Study the drawing (mm; zero at the part's minimum x, y, z) and answer. A direction names the side the tool comes from. Coordinates: 2 decimals unless noted, no trailing zeros. Loops run counter-clockwise (first coordinate to the right, second up) from the corner with the lowest first, then second, coordinate; pieces in that order, holes last. Notation, with made-up numbers: (-13, -21) - (38, -21) arc R21 cw to (38, 10) - close; hole circle Ø2 at (-19.5, -19.5). An arc over 180 degrees is marked (long way). Use one line per item in the form item = value.
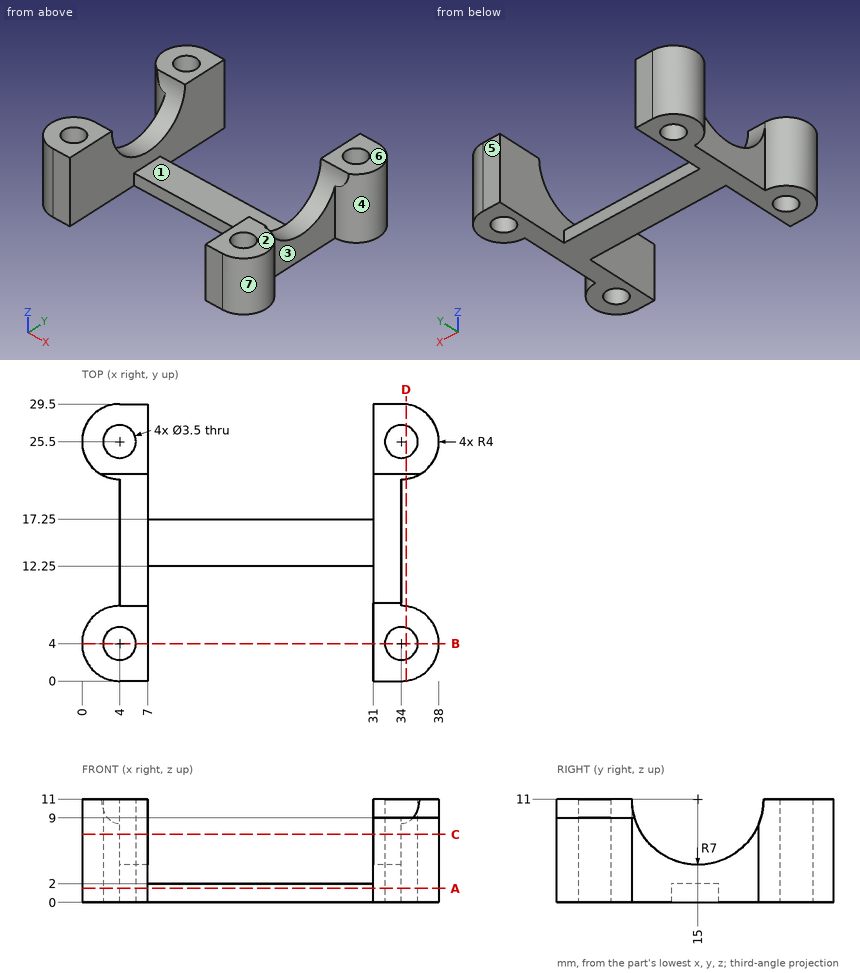
Item 1: The part is cut by section B-B on y = 4. Give the vertices of the cut face in (x, z).
Results below:
outline = (0, 0) - (2.25, 0) - (2.25, 11) - (0, 11) - close; (5.75, 0) - (7, 0) - (7, 11) - (5.75, 11) - close; (31, 0) - (32.25, 0) - (32.25, 9) - (31, 9) - close; (35.75, 0) - (38, 0) - (38, 9) - (35.75, 9) - close
Item 2: Which of the six approach directions +Z, -Z, +X, -X, +Y, -Y give full straight-line access (tool end or side, diameter ignored) to the marked faces 1, 2 and 3?
Results below:
face_1 = +Z, +Y, -Y
face_2 = +Z, +X, -Y
face_3 = +Z, -Z, +X
Item 3: The part is cut by section A-A on z = 1.5. Give the vertices of the cut face in (x, y), plus the area to 3 significant figures.
Results below:
outline = (4, 0) - (7, 0) - (7, 12.25) - (31, 12.25) - (31, 0) - (34, 0) arc R4 ccw to (34, 8) - (34, 21.5) arc R4 ccw to (34, 29.5) - (31, 29.5) - (31, 17.25) - (7, 17.25) - (7, 29.5) - (4, 29.5) arc R4 ccw to (4, 21.5) - (4, 8) arc R4 ccw to start; hole circle Ø3.5 at (4, 4); hole circle Ø3.5 at (4, 25.5); hole circle Ø3.5 at (34, 4); hole circle Ø3.5 at (34, 25.5)
area = 359 mm²
Item 4: Find the intervals of material crossed by L1, parallel to X at y = 26.75, z = 2; L2, parallel to Y at x = 33.5, z = 2.5; L3, parallel to Y at x = 35, z = 3, in increasing order.
Results below:
L1 = 0.2 to 2.78, 5.22 to 7, 31 to 32.78, 35.22 to 37.8
L2 = 0 to 2.32, 5.68 to 23.82, 27.18 to 29.5
L3 = 0.13 to 2.56, 5.44 to 7.87, 21.63 to 24.06, 26.94 to 29.37
Item 5: For a pull along Y with two mould halves and no side action, classify the marked faces 4, 5, 6 and 7 as +Y half, -Y half, draft (parallel to the pull), parting line (faces both ways), or undercut.
Results below:
face_4 = undercut
face_5 = +Y half
face_6 = draft
face_7 = undercut
Item 6: The part is cut by section D-D on x = 34.5. Give the vertices of the cut face in (y, z).
Results below:
outline = (0.03, 0) - (2.32, 0) - (2.32, 9) - (0.03, 9) - close; (5.68, 0) - (7.97, 0) - (7.97, 9) - (5.68, 9) - close; (21.53, 0) - (23.82, 0) - (23.82, 11) - (22, 11) arc R7 cw to (21.53, 8.48) - close; (27.18, 0) - (29.47, 0) - (29.47, 11) - (27.18, 11) - close
Item 7: The part is cut by section C-C on z = 7.25. Give the vertices of the cut face in (x, y), plus the area to 3 significant figures.
Results below:
outline = (4, 0) - (7, 0) - (7, 9.09) - (4, 9.09) - (4, 8) arc R4 ccw to start; (4, 20.91) - (7, 20.91) - (7, 29.5) - (4, 29.5) arc R4 ccw to (4, 21.5) - close; (31, 0) - (34, 0) arc R4 ccw to (34, 8) - (34, 9.09) - (31, 9.09) - close; (31, 20.91) - (34, 20.91) - (34, 21.5) arc R4 ccw to (34, 29.5) - (31, 29.5) - close; hole circle Ø3.5 at (4, 4); hole circle Ø3.5 at (4, 25.5); hole circle Ø3.5 at (34, 4); hole circle Ø3.5 at (34, 25.5)
area = 168 mm²
Item 8: Each of these flat-tipped pins is pushed along its axis until it touches: P1, Ø3, axis at x = 10, z = 6, coming from the -Y side; P2, Ø2.5, axis at y = 14.5, z = 3, coming from the +X side; P3, Ø0.6, axis at x = 21, z = 1.5, coming from the +Y side; P4, Ø5.5, axis at x = 16.5, y = 14, coming from the +Z side. Where does it stop, or does it pass through?
Results below:
P1 = through
P2 = 34
P3 = 17.25
P4 = 2
